Here's how the part is built. I have some questions about the finished solid (model axes, mm). Face numbers are marked on the shaded views. A direction names the side the tool comes from. Give positions to 0.01 mm unless a question says otherwise; leave off trailing zeros. Order: outer loops, then holes, each group sorted by start corner. A loop starts at its lowest first (then second) coordinate and runs counter-clockwise, first axis right, second up. Notation, with made-up numbers: M 42,-0.5 L 54,-0.5 A19 ccw 54,18.5 Z; hole C 81.5,52.25 d1. An arc over 180 degrees is marked long. Use CSV: the item, a comma, the result in double quotes. Start each with the question number.
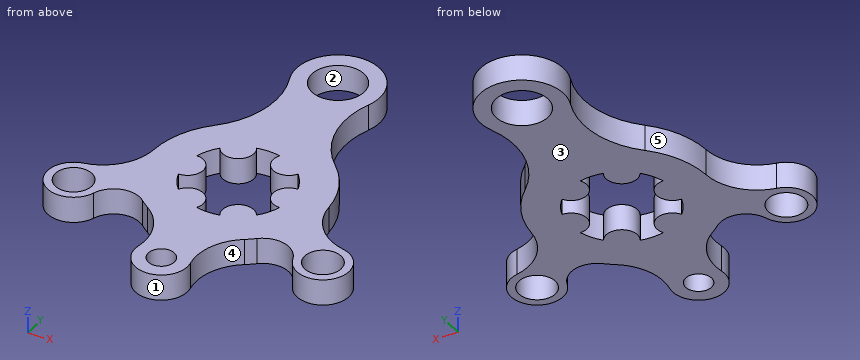
```python
from build123d import *

# Parameters (mm, degrees)
SKETCH1_R           = 7
SKETCH1_R_2         = 5
SKETCH1_R_3         = 10
BOSS_EXTRUDE1_DEPTH = 10


with BuildPart() as part:
    # Sketch1 → Boss-Extrude1 (new body)
    with BuildSketch(Plane.XY):
        with BuildLine():
            ThreePointArc((-14.869403875, 59.092307692), (-13.366464174, 40.352096999), (-22.647245902, 24.002130178))
            ThreePointArc((-22.647245902, 24.002130178), (-29.864288772, 14.040094593), (-32.931378534, 2.127042038))
            ThreePointArc((-32.931378534, 2.127042038), (-37.838433301, -9.754136505), (-48.963263256, -16.194613858))
            ThreePointArc((-48.963263256, -16.194613858), (-54.534765397, -32.574747935), (-37.550915036, -29.273345896))
            ThreePointArc((-37.550915036, -29.273345896), (-30.697148757, -22.889346352), (-21.566520754, -24.9776937))
            ThreePointArc((-21.566520754, -24.9776937), (-19.978209416, -26.265398313), (-18.313197236, -27.452264151))
            ThreePointArc((-18.313197236, -27.452264151), (-10.929939867, -36.447383635), (-9.804034884, -48.03))
            ThreePointArc((-9.804034884, -48.03), (0, -60), (9.804034884, -48.03))
            ThreePointArc((9.804034884, -48.03), (10.929939867, -36.447383635), (18.313197236, -27.452264151))
            ThreePointArc((18.313197236, -27.452264151), (19.978209416, -26.265398313), (21.566520754, -24.9776937))
            ThreePointArc((21.566520754, -24.9776937), (30.697148757, -22.889346352), (37.550915036, -29.273345896))
            ThreePointArc((37.550915036, -29.273345896), (54.534765397, -32.574747935), (48.963263256, -16.194613858))
            ThreePointArc((48.963263256, -16.194613858), (37.838433301, -9.754136505), (32.931378534, 2.127042038))
            ThreePointArc((32.931378534, 2.127042038), (29.864288772, 14.040094593), (22.647245902, 24.002130178))
            ThreePointArc((22.647245902, 24.002130178), (13.366464174, 40.352096999), (14.869403875, 59.092307692))
            ThreePointArc((14.869403875, 59.092307692), (0, 81), (-14.869403875, 59.092307692))
        make_face()
        with Locations((-47, -26)):
            Circle(SKETCH1_R, mode=Mode.SUBTRACT)
        with Locations((0, -50)):
            Circle(SKETCH1_R_2, mode=Mode.SUBTRACT)
        with Locations((47, -26)):
            Circle(SKETCH1_R, mode=Mode.SUBTRACT)
        with BuildLine():
            ThreePointArc((-14.735544437, -13.522711642), (-17.320508076, -10), (-19.078784028, -6))
            ThreePointArc((-19.078784028, -6), (-13.078784028, 0), (-19.078784028, 6))
            ThreePointArc((-19.078784028, 6), (-17.320508076, 10), (-14.735544437, 13.522711642))
            ThreePointArc((-14.735544437, 13.522711642), (-6.539392014, 11.326559219), (-4.343239591, 19.522711642))
            ThreePointArc((-4.343239591, 19.522711642), (0, 20), (4.343239591, 19.522711642))
            ThreePointArc((4.343239591, 19.522711642), (6.539392014, 11.326559219), (14.735544437, 13.522711642))
            ThreePointArc((14.735544437, 13.522711642), (17.320508076, 10), (19.078784028, 6))
            ThreePointArc((19.078784028, 6), (13.078784028, 0), (19.078784028, -6))
            ThreePointArc((19.078784028, -6), (17.320508076, -10), (14.735544437, -13.522711642))
            ThreePointArc((14.735544437, -13.522711642), (6.539392014, -11.326559219), (4.343239591, -19.522711642))
            ThreePointArc((4.343239591, -19.522711642), (0, -20), (-4.343239591, -19.522711642))
            ThreePointArc((-4.343239591, -19.522711642), (-6.539392014, -11.326559219), (-14.735544437, -13.522711642))
        make_face(mode=Mode.SUBTRACT)
        with Locations((0, 65)):
            Circle(SKETCH1_R_3, mode=Mode.SUBTRACT)
    extrude(amount=BOSS_EXTRUDE1_DEPTH)


solid = part.part
```
Q1. Imagine slicing it at A-A, the plane y = 65. Please give me the cut outline in (x, z), then the cut area to 3 significant figures.
Q2. I need wall thicknesses on line 1 (Y direction, x = 0, z = 3); line 2 (Y direction, x = -41, z = 5.5); line 3 (Y direction, x = -47, z = 6.25). Which ranges of each line are inside material? Lowest first, please. Write a range as [from, to].
Q3. Imagine slicing it at B-B, the plane x = 47. Please give me the cut outline in (y, z), then the cut area to 3 significant figures.
Q4. For the marked faces 4 and 5, which set-ups out of +Z, -Z, +X, -X, +Y, -Y let a thin tool reach every point of the face, with its end or its side?
Q5. We'd pull the mould along X, two halves only. Please class the marked faces 1, 2 and 3: pulls with the +X half, pulls with the -X half, needs draft (parallel to the pull), parting line crosses it, or undercut.
Q6. For P1, Ø16, axis at x = 0, y = 65, coming from the +Z side; P2, Ø4, axis at y = 26, z = 8.5, coming from the +X side; P3, Ø6, axis at y = 36.5, z = 3, coming from the +X side; P4, Ø3, axis at y = 66, z = 6.5, coming from the -X side, each with a flat end and sliding along its axis, tell me the tip position at first contact or that it passes through.
Q7. Imagine slicing it at D-D, the plane x = 29.5. Please give me the cut outline in (y, z), then the cut area to 3 significant figures.
Q8. Imagine slicing it at C-C, the plane z = 7. Count the separate pieces of the cut face and the enclosed holes in it, then the cut area to 3 significant figures.
Reply:
1,outline,"M -16,0 L -10,0 L -10,10 L -16,10 Z; M 10,0 L 16,0 L 16,10 L 10,10 Z"
1,area,"120 mm^2"
2,line 1,"y = [-60, -55], [-45, -20], [20, 55], [75, 81]"
2,line 2,"y = [-34, -29.61], [-22.39, -12.67]"
2,line 3,"y = [-36, -33], [-19, -15.7]"
3,outline,"M -36,0 L -33,0 L -33,10 L -36,10 Z; M -19,0 L -15.7,0 L -15.7,10 L -19,10 Z"
3,area,"63.0 mm^2"
4,face 4,"+Z, -Z"
4,face 5,"+Z, -Z, -X, +Y"
5,face 1,"parting line crosses it"
5,face 2,"undercut"
5,face 3,"needs draft"
6,P1,"passes through"
6,P2,"stops at x = 22.65"
6,P3,"stops at x = 15.73"
6,P4,"stops at x = -16"
7,outline,"M -22.64,0 L 14.79,0 L 14.79,10 L -22.64,10 Z"
7,area,"374 mm^2"
8,separate pieces,"1"
8,enclosed holes,"5"
8,area,"4,770 mm^2"
